The model under review builds one solid part; all positions refer to its coordinate system, in mm. Round coordinates to 2 decimals unless told otherwise and drop trailing zeros. Loops run counter-clockwise (first coordinate to the right, second up) from the corner with the lowest first, then second, coordinate; pieces in that order, holes last. Notation, with made-up numbers: (35.25, -5.75) -> (65.25, -5.75) arc R18 cw to (65.25, 28.25) -> close; hole circle Ø10 at (77, -25). An arc over 180 degrees is marked (long way). Use a Markdown table: item, result. Add a question column.
1) Consider section A-A on x = 109.5. Give the boundary of the cut face in (y, z), plus the area to 3 significant figures.
2) Wall thickness on probe 1 along Y at (x, z) = (63, 1.6); probe 2 along Y at (x, z) = (108, 2.7); probe 3 along Y at (x, z) = (102, 1.15): over which ranges is each line inside the solid? List them lowest first.
3) Consider section D-D on x = 138.5. Give the boundary of the cut face in (y, z).
4) Insertion check: pin 1 (0.9 mm diameter, centred on y = 81, z = 2, fed in from +X). The pin has a flat end and moves straight along its axis. Give the tip position at first contact, or say it passes through.
5) Consider section C-C on x = 97. Give the boundary of the cut face in (y, z), plus the area to 3 significant figures.
6) Consider section B-B on z = 1.85. Give the boundary of the cut face in (x, y).
from build123d import *

# Parameters (mm, degrees)
MODEL_R                 = 6
MODEL_W                 = 24
MODEL_H                 = 3
SALIENTE_EXTRUIR1_DEPTH = 3


with BuildPart() as part:
    # Model → Saliente-Extruir1 (new body)
    with BuildSketch(Plane.XY):
        Polygon((54, 89), (54, 81.9), (65.8, 81.9), (65.8, 58.7), (54, 58.7), (54, -69), (146, -69), (146, 58.7), (134.2, 58.7), (134.2, 81.9), (146, 81.9), (146, 89), align=None)
        with Locations((99.899304233, 61.529562992)):
            Circle(MODEL_R, mode=Mode.SUBTRACT)
        with Locations((100, 80.5)):
            Rectangle(MODEL_W, MODEL_H, mode=Mode.SUBTRACT)
    extrude(amount=SALIENTE_EXTRUIR1_DEPTH)


solid = part.part
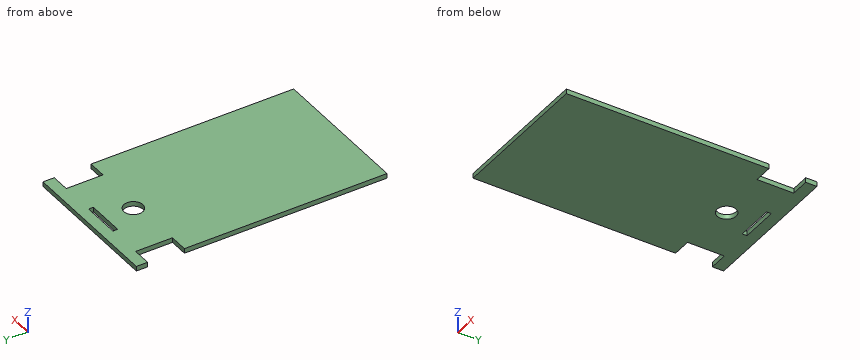
Result set:
| question | item | result |
|---|---|---|
| 1 | outline | (-69, 0) -> (79, 0) -> (79, 3) -> (-69, 3) -> close; (82, 0) -> (89, 0) -> (89, 3) -> (82, 3) -> close |
| 1 | area | 465 mm2 |
| 2 | probe 1 | -69 to 58.7, 81.9 to 89 |
| 2 | probe 2 | -69 to 79, 82 to 89 |
| 2 | probe 3 | -69 to 55.91, 67.15 to 79, 82 to 89 |
| 3 | outline | (-69, 0) -> (58.7, 0) -> (58.7, 3) -> (-69, 3) -> close; (81.9, 0) -> (89, 0) -> (89, 3) -> (81.9, 3) -> close |
| 4 | pin 1 | x = 134.2 |
| 5 | outline | (-69, 0) -> (56.28, 0) -> (56.28, 3) -> (-69, 3) -> close; (66.78, 0) -> (79, 0) -> (79, 3) -> (66.78, 3) -> close; (82, 0) -> (89, 0) -> (89, 3) -> (82, 3) -> close |
| 5 | area | 433 mm2 |
| 6 | outline | (54, -69) -> (146, -69) -> (146, 58.7) -> (134.2, 58.7) -> (134.2, 81.9) -> (146, 81.9) -> (146, 89) -> (54, 89) -> (54, 81.9) -> (65.8, 81.9) -> (65.8, 58.7) -> (54, 58.7) -> close; hole (88, 79) -> (112, 79) -> (112, 82) -> (88, 82) -> close; hole circle Ø12 at (99.9, 61.53) |
